Autodesk Inventor part; units mm, degrees
ref_plane "Work Plane1" through (31.775, 0, -7.95) normal (0, 0, -1) x (-1, 0, 0)
ref_plane "YZ Plane" through (0, 0, 0) normal (1, 0, 0) x (0, 1, 0)
ref_plane "XZ Plane" through (0, 0, 0) normal (0, 1, 0) x (-1, 0, 0)
ref_plane "Work Plane1" through (31.775, 0, -7.95) normal (0, 0, -1) x (-1, 0, 0)
sketch "Sketch1" plane through (31.775, 0, -7.95) normal (0, 0, -1) x (-1, 0, 0)
  line L0 (62.5134, -8.05) -> (55.6, -8.05) construction
  line L1 (55.6, -8.05) -> (55.6, 8.05) construction
  line L2 (55.6, 8.05) -> (62.5134, 8.05) construction
  arc A0 (62.5134, 8.05) -> (1.0366, 8.05) centre (31.775, 0) ccw construction
  line L3 (1.0366, 8.05) -> (7.95, 8.05) construction
  line L4 (7.95, 8.05) -> (7.95, -8.05) construction
  line L5 (7.95, -8.05) -> (1.0366, -8.05) construction
  arc A1 (1.0366, -8.05) -> (62.5134, -8.05) centre (31.775, 0) ccw construction
  circle A2 centre (31.775, 0) radius 22.225 construction
  circle A3 centre (31.775, 0) radius 22.325
  line L6 (69.275, 37.5) -> (-5.725, 37.5)
  line L7 (-5.725, 37.5) -> (-5.725, -37.5)
  line L8 (-5.725, -37.5) -> (69.275, -37.5)
  line L9 (69.275, -37.5) -> (69.275, 37.5)
  line L10 (69.275, 37.5) -> (-5.725, -37.5) construction
  line L11 (-5.725, 37.5) -> (69.275, -37.5) construction
  dimension "d0" = 0.1
  dimension "d1" = 44.65
  dimension "d2" = 75
extrude "Extrusion1" add sketch "Sketch1" along normal blind 8
sketch "Sketch2" plane through (31.775, 0, -7.95) normal (0, 0, 1) x (1, 0, 0)
  line L0 (-62.5134, -8.05) -> (-55.6, -8.05) construction
  line L1 (-55.6, -8.05) -> (-55.6, 8.05) construction
  line L2 (-55.6, 8.05) -> (-62.5134, 8.05) construction
  arc A0 (-1.0366, 8.05) -> (-62.5134, 8.05) centre (-31.775, 0) ccw construction
  line L3 (-1.0366, 8.05) -> (-7.95, 8.05) construction
  line L4 (-7.95, 8.05) -> (-7.95, -8.05) construction
  line L5 (-7.95, -8.05) -> (-1.0366, -8.05) construction
  arc A1 (-62.5134, -8.05) -> (-1.0366, -8.05) centre (-31.775, 0) ccw construction
  circle A2 centre (-31.775, 0) radius 22.225 construction
  line L6 (5.725, 37.5) -> (5.725, -37.5)
  line L7 (-69.275, 37.5) -> (5.725, 37.5)
  line L8 (-69.275, -37.5) -> (-69.275, 37.5)
  line L9 (5.725, -37.5) -> (-69.275, -37.5)
  circle A3 centre (-31.775, 0) radius 22.325 construction
  circle A4 centre (-31.775, 0) radius 31.875
  line L10 (-55.6, -8) -> (-69.275, -8)
  line L11 (-69.275, -8) -> (-69.275, 8)
  line L12 (-69.275, 8) -> (-55.6, 8)
  line L13 (-55.6, 8) -> (-55.6, -8)
  line L14 (-84.275, 0) -> (20.725, 0) construction
  line L15 (-31.775, -52.5) -> (-31.775, 52.5) construction
  line L16 (-1.0366, -8.05) -> (-7.95, -8.05) construction
  line L17 (-7.95, -8.05) -> (-7.95, 8.05) construction
  line L18 (-7.95, 8.05) -> (-1.0366, 8.05) construction
  line L19 (-7.95, -8) -> (5.725, -8)
  line L20 (5.725, -8) -> (5.725, 8)
  line L21 (5.725, 8) -> (-7.95, 8)
  line L22 (-7.95, 8) -> (-7.95, -8)
  point P0 (-62.6298, 8)
  point P1 (-62.6298, -8)
  point P2 (-0.9202, 8)
  point P3 (5.725, 8)
  point P4 (5.725, -8)
  point P5 (-0.9202, -8)
  dimension "d7" = 0.1
  dimension "d9" = 0
  dimension "d29" = 0.05
extrude "Extrusion2" add sketch "Sketch2" along normal blind 15 contours L6 L21 A4 L12 L8 L7 | L6 L9 L8 L10 A4 L19
sketch "Sketch3" plane through (31.775, 0, 7.05) normal (0, 0, 1) x (1, 0, 0)
  line L0 (-3.025, -28.75) -> (-60.525, -28.75)
  line L1 (-60.525, -28.75) -> (-60.525, 28.75)
  line L2 (-60.525, 28.75) -> (-3.025, 28.75)
  line L3 (-3.025, 28.75) -> (-3.025, -28.75)
  line L4 (-3.025, -28.75) -> (-60.525, 28.75) construction
  line L5 (-60.525, -28.75) -> (-3.025, 28.75) construction
  point P0 (-31.775, 0)
  dimension "d12" = 57.5
hole "Hole1" at (-28.75, 28.75, 7.05) at (28.75, 28.75, 7.05) at (28.75, -28.75, 7.05) at (-28.75, -28.75, 7.05) direction (0, 0, -1) diameter 6.5 end through all counterbore diameter 12 counterbore depth 12
sketch "Sketch4" plane through (31.775, 0, -7.95) normal (0, 0, 1) x (1, 0, 0)
  circle A0 centre (-31.775, 0) radius 22.325 construction
  line L0 (5.725, 8) -> (-0.9202, 8) construction
  arc A1 (-0.9202, 8) -> (-62.6298, 8) centre (-31.775, 0) ccw construction
  line L1 (-62.6298, 8) -> (-69.275, 8) construction
  line L2 (-69.275, -8) -> (-69.275, 8) construction
  line L3 (-69.275, -8) -> (-62.6298, -8) construction
  arc A2 (-62.6298, -8) -> (-0.9202, -8) centre (-31.775, 0) ccw construction
  line L4 (-0.9202, -8) -> (5.725, -8) construction
  line L5 (5.725, 8) -> (5.725, -8) construction
  line L6 (5.725, 8) -> (-7.95, 8) construction
  line L7 (-7.95, -8) -> (5.725, -8) construction
  line L8 (5.725, -8) -> (5.725, 8) construction
  line L9 (-31.775, 0) -> (-9.45, 0) construction
  line L10 (-9.45, 0) -> (5.725, 0) construction
  line L11 (-1.1125, 8) -> (-1.1125, -8) construction
  line L12 (-0.9202, -8) -> (5.725, -8) construction
  line L13 (-31.775, -52.5) -> (-31.775, 52.5) construction
  line L14 (-7.95, -8) -> (-7.95, 8)
  line L15 (-7.95, 8.05) -> (-7.95, -8.05)
  point P0 (-1.1125, 0)
  point P1 (-62.4375, 0)
  dimension "d28" = 0
hole "Hole2" at (30.6625, 0, -7.95) at (-30.6625, 0, -7.95) direction (0, 0, -1) diameter 4.134 end through all countersink diameter 6.5 countersink angle 90
fillet "Fillet1" radius 8 4 edges at (-37.5, -37.5, -4.45) (-37.5, 37.5, -4.45) (37.5, 37.5, -4.45) (37.5, -37.5, -4.45)
chamfer "Chamfer1" distance 1.5 angle 45 16 edges at (0, 31.875, 7.05) (0, -31.875, 7.05) (34.1774, 8, 7.05) (-34.1774, 8, 7.05) (-34.1774, -8, 7.05) (-37.5, -18.75, 7.05) (-35.1569, -35.1569, 7.05) (0, -37.5, 7.05) (35.1569, -35.1569, 7.05) (37.5, -18.75, 7.05) (-37.5, 18.75, 7.05) (-35.1569, 35.1569, 7.05) (0, 37.5, 7.05) (35.1569, 35.1569, 7.05) (37.5, 18.75, 7.05) (34.1774, -8, 7.05)
chamfer "Chamfer2" distance 1 angle 45 1 edges at (22.325, 0, -7.95)
chamfer "Chamfer3" distance 0.5 angle 45 6 edges at (30.6625, 2.067, -15.95) (-30.6625, 2.067, -15.95) (28.75, -25.5, -15.95) (-28.75, -25.5, -15.95) (28.75, 32, -15.95) (-28.75, 32, -15.95)
chamfer "Chamfer5" distance 0.5 angle 45 8 edges at (-30.8548, 8, -1.2) (30.8548, 8, -1.2) (-30.8548, -8, -1.2) (30.8548, -8, -1.2) (-37.5, 8, -1.2) (37.5, 8, -1.2) (37.5, -8, -1.2) (-37.5, -8, -1.2)
properties part number "TH1-001" material "Aluminum 6061"
Geometry: final body of the model. Coordinates: model frame, mm. A direction names the side the tool comes from. Coordinates: 2 decimals unless noted, no trailing zeros. Loops run counter-clockwise (first coordinate to the right, second up) from the corner with the lowest first, then second, coordinate; pieces in that order, holes last. Notation, with made-up numbers: M 22.5,-26 L 71.5,-26 A24 cw 71.5,-2 Z; hole C 2,30.25 d4. An arc over 180 degrees is marked long. One line per item, written item: value. Start each with the question number.
1) Material intervals for L1, parallel to Y at x = -28.75, z = 0.5; L2, parallel to X at y = -28.75, z = -11, sorted ascending. Write a range as from..to.
2) Cut plane B-B (x = 0). Return loops of the section in (y, z) (3 decimals), then the cut area to 3 significant figures.
3) Reachability of faces 5 (the cylindrical face through (35.094, -35.219, -5.049)), 6 (the cylindrical face through (32.4, -23.99, 0.97)), 7 (the flat face through (-34, 8, -1)) from +Z, -Z, +X, -X, +Y, -Y: full face, straight path, thin tool, end or side. Return the list, or none.
4) Pin query (flat end, axial travel): P1, Ø7, axis at x = 28.75, y = -28.75, coming from the -Z side; P2, Ø1.7, axis at x = -34, z = -3, coming from the +Y side; P3, Ø6, axis at x = 33, z = 0.5, coming from the +Y side; P4, Ø9.5, axis at x = -26.5, y = -31, coming from the +Z side. Return the tip coordinate at first contact, or that it passes through.
5) Cut plane C-C (z = -10.25). Count the separate pieces of the cut face and the enclosed holes in it, then the cut area to 3 significant figures.
6) Draft query along Y for faces 1 (the conical face through (34.344, 34.452, 6.623)), 2 (the cylindrical face through (-35.219, -35.094, -5.049)), 3 (the cylindrical face through (-28.645, 0.448, -12.336)), 4 (the flat face through (17, -16, -15.95)). Return one class per face: released by +Y, released by -Y, zero draft, split by the parting line, or undercut.
7) Cut plane A-A (z = 3.75). Return loops of the section in (x, y) (3 decimals), then the cut area to 3 significant figures.
Evaluation:
1. L1: -37.5..-34.75, -22.75..-13.76, 13.76..22.75, 34.75..37.5
1. L2: -37.5..-32, -25.5..25.5, 32..37.5
2. outline: M -37.5,-15.95 L -22.325,-15.95 L -22.325,-8.95 L -23.325,-7.95 L -31.875,-7.95 L -31.875,5.55 L -33.375,7.05 L -36,7.05 L -37.5,5.55 Z; M 22.325,-15.95 L 37.5,-15.95 L 37.5,5.55 L 36,7.05 L 33.375,7.05 L 31.875,5.55 L 31.875,-7.95 L 23.325,-7.95 L 22.325,-8.95 Z
2. area: 406 mm^2
3. face 5: +Z, -Z, +X, -Y
3. face 6: +Z
3. face 7: +Z, +X, -X
4. P1: z = -15.7
4. P2: y = 36.62
4. P3: y = 37.48
4. P4: z = 7.05
5. separate pieces: 1
5. enclosed holes: 7
5. area: 3,840 mm^2
6. face 1: released by +Y
6. face 2: released by -Y
6. face 3: undercut
6. face 4: zero draft
7. outline: M -37.5,-29.5 A8 ccw -29.5,-37.5 L 29.5,-37.5 A8 ccw 37.5,-29.5 L 37.5,-8.5 L 37,-8 L 31.355,-8 L 30.725,-8.483 A31.875 cw -30.725,-8.483 L -31.355,-8 L -37,-8 L -37.5,-8.5 Z; M -37.5,8.5 L -37,8 L -31.355,8 L -30.725,8.483 A31.875 cw 30.725,8.483 L 31.355,8 L 37,8 L 37.5,8.5 L 37.5,29.5 A8 ccw 29.5,37.5 L -29.5,37.5 A8 ccw -37.5,29.5 Z; hole C -28.75,-28.75 d12; hole C -28.75,28.75 d12; hole C 28.75,-28.75 d12; hole C 28.75,28.75 d12
7. area: 1,730 mm^2
